from build123d import *

# Parameters (mm, degrees)
SKETCH1_W           = 19.53
SKETCH1_H           = 19.278
BOSS_EXTRUDE1_DEPTH = 5.85
SKETCH2_W           = 4
SKETCH2_H           = 3
BOSS_EXTRUDE2_DEPTH = 5.85
CAVITY1_START       = -3.175
CAVITY1_OUTLINE_W   = 5.85
CAVITY1_OUTLINE_H   = 12.778
CAVITY1_DEPTH       = 6.35


# Read off the part's stored shape, not the designer's step: Cavity1
with BuildPart() as part:
    # Sketch1 → Boss-Extrude1 (new body)
    with BuildSketch(Plane(origin=(0, 0, 0), x_dir=(1, 0, 0), z_dir=(0, 1, 0))):
        Rectangle(SKETCH1_W, SKETCH1_H)
    extrude(amount=BOSS_EXTRUDE1_DEPTH)

    # Sketch2 → Boss-Extrude2 (add)
    with BuildSketch(Plane(origin=(0, 5.85, 0), x_dir=(1, 0, 0), z_dir=(0, 1, 0))):
        with Locations((-7.765, 11.139)):
            Rectangle(SKETCH2_W, SKETCH2_H)
        with Locations((7.765, 11.139)):
            Rectangle(SKETCH2_W, SKETCH2_H)
    extrude(amount=-BOSS_EXTRUDE2_DEPTH)

    # Cavity1 outline → Cavity1 (cut)
    with BuildSketch(Plane.YZ.offset(CAVITY1_START)):
        with Locations((2.925, 3.25)):
            Rectangle(CAVITY1_OUTLINE_W, CAVITY1_OUTLINE_H)
    extrude(amount=CAVITY1_DEPTH, mode=Mode.SUBTRACT)


solid = part.part
Design review of the part built by this model. Coordinates are the model's own, in mm. A direction names the side the tool comes from. Round coordinates to 2 decimals unless told otherwise and drop trailing zeros. Loops run counter-clockwise (first coordinate to the right, second up) from the corner with the lowest first, then second, coordinate; pieces in that order, holes last. Notation, with made-up numbers: (-31.75, -10) -> (-5.75, -10) arc R23 ccw to (-5.75, 18) -> close; hole circle Ø5 at (32, 86.25). An arc over 180 degrees is marked (long way). Use one line per item in the form item = value. Start each with the question number.
Q1. We need section C-C on x = -1.5. Give the boundary of the cut face in (y, z), then the cut area to 3 significant figures.
Q2. Machinability: for faces 1 (the face through (0, 3, -3.139)), 2 (the face through (0, 5.85, -4)), 3 (the face through (0, 3, -9.639)), which of the approach directions +Z, -Z, +X, -X, +Y, -Y give a long, thin tool a straight path to every point of the face, cutting with its end or side? Answer none if there is none.
Q3. Draft analysis for pull direction X (two halves, no side actions). For faces 4 (the face through (8, 3, -12.639)), 5 (the face through (5.765, 3, -11)), 6 (the face through (-9.765, 3, -1)), 7 (the face through (9.765, 3, -1)), state which applies: +X half, -X half, draft (parallel to the pull), parting line (faces both ways), or undercut.
Q4. Wall thickness on line 1 along X through (y, z) = (4.35, -11.5) (3 decimals); line 2 along X through (y, z) = (3.05, 3) (3 decimals); line 3 along Z through (x, y) = (-1.5, 5.2): over which ranges is each line inside the solid? List them lowest first. Write a range as [from, to].
Q5. For pin 1 Ø1 at (x, y) = (-2.5, 4.5) entering from -Z; pin 2 Ø3 at (x, y) = (-0.5, 2) entering from +Z; pin 3 Ø3 at (x, z) = (-0.5, 4) entering from +Y, all flat-tipped, find the tip position at first contact; note any pin that passes through.
Q6. We need section B-B on y = 4.2. Give the boundary of the cut face in (x, z) (3 decimals).
Q7. We need section A-A on z = -0.25. Give the boundary of the cut face in (x, y) (3 decimals), then the cut area to 3 significant figures.
Calculated:
q1.outline = (0, -9.64) -> (5.85, -9.64) -> (5.85, -3.14) -> (0, -3.14) -> close
q1.area = 38.0 mm²
q2.face_1 = +Z, +Y, -Y
q2.face_2 = +Z, -Z, +X, -X, +Y
q2.face_3 = -Z, +Y, -Y
q3.face_4 = draft
q3.face_5 = undercut
q3.face_6 = -X half
q3.face_7 = +X half
q4.line_1 = [-9.765, -5.765], [5.765, 9.765]
q4.line_2 = [-9.765, -3.175], [3.175, 9.765]
q4.line_3 = [-9.64, -3.14]
q5.pin_1 = -9.64
q5.pin_2 = -3.14
q5.pin_3 = through
q6.outline = (-9.765, -12.639) -> (-5.765, -12.639) -> (-5.765, -9.639) -> (5.765, -9.639) -> (5.765, -12.639) -> (9.765, -12.639) -> (9.765, 9.639) -> (3.175, 9.639) -> (3.175, -3.139) -> (-3.175, -3.139) -> (-3.175, 9.639) -> (-9.765, 9.639) -> close
q7.outline = (-9.765, 0) -> (-3.175, 0) -> (-3.175, 5.85) -> (-9.765, 5.85) -> close; (3.175, 0) -> (9.765, 0) -> (9.765, 5.85) -> (3.175, 5.85) -> close
q7.area = 77.1 mm²
